Check sheet for the modelled part. Datum: model origin and axes. Units: mm. A direction names the side the tool comes from. Round coordinates to 2 decimals unless told otherwise and drop trailing zeros. Loops run counter-clockwise (first coordinate to the right, second up) from the corner with the lowest first, then second, coordinate; pieces in that order, holes last. Notation, with made-up numbers: (52, 85) -> (70, 85) arc R38 ccw to (70, 124) -> close; hole circle Ø6 at (43.25, 88). An arc over 180 degrees is marked (long way). One line per item, written item: value. Start each with the question number.
1. Material ranges on L1, parallel to X at y = 11, z = 5.75; L2, parallel to Y at x = -0.5, z = 4.5; L3, parallel to Y at x = 56, z = 0.75, recorded low to high.
2. Set-up check for faces 4 (the face through (-49.01, -42.45, 3.22)), 5 (the face through (-117.614, -82.61, 3.219)): record each of +Z, -Z, +X, -X, +Y, -Y from which the full face is reachable in a straight line by a thin tool's end or side.
3. Release check for a two-part mould opening along Y. For faces 1 (the face through (-16.45, 53.61, 3.22)), 2 (the face through (-117.614, 82.61, 3.219)), 3 (the face through (117.535, -82.689, 3.219)) record: +Y half, -Y half, draft (parallel to the pull), parting line (faces both ways), or undercut.
4. Cross-section at C-C on y = 50.5. Record the cut outline in (x, z).
5. Cross-section at B-B on x = -54.5. Record the cut outline in (y, z), then the cut area to 3 significant figures.
6. Cross-section at A-A on z = 5.25. Record the cut outline in (x, y) (1 decimal), then the cut area to 3 significant figures.
from build123d import *

# Parameters (mm, degrees)
F0_W     = 238.125
F0_H     = 168.275
F1_DEPTH = 6.35
F2_R     = 5.08
F4_DEPTH = 25.4
F5_DEPTH = 6.351
F7_DEPTH = 6.351


with BuildPart() as f1:
    # F0 (on Top) → F1 (new body)
    with BuildSketch(Plane.XY):
        Rectangle(F0_W, F0_H)
    extrude(amount=F1_DEPTH)

    # F2
    f2_edges = [f1.edges().sort_by_distance(p)[0] for p in [
        (-119.0625, 84.1375, 3.175),
        (119.0625, 84.1375, 3.175),
        (-119.0625, -84.1375, 3.175),
        (119.0625, -84.1375, 3.175),
    ]]
    fillet(f2_edges, radius=F2_R)

    # F3 (on face) → F4 (cut)
    with BuildSketch(Plane.XY.offset(6.35)):
        Polygon((-63.5, -58.7375), (0, -58.7375), (63.5, -58.7375), (31.75, -26.9875), (31.75, 36.5125), (0, 68.2625), (-31.75, 36.5125), (-31.75, -26.9875), align=None)
    extrude(amount=-F4_DEPTH, mode=Mode.SUBTRACT)

    # F3 (on face) → F5 (cut, through all)
    with BuildSketch(Plane.XY.offset(6.35)):
        Polygon((-63.5, -58.7375), (0, -58.7375), (63.5, -58.7375), (31.75, -26.9875), (31.75, 36.5125), (0, 68.2625), (-31.75, 36.5125), (-31.75, -26.9875), align=None)
    extrude(amount=-F5_DEPTH, mode=Mode.SUBTRACT)

    # F6 (on face) → F7 (cut, through all)
    with BuildSketch(Plane.XY.offset(6.35)):
        with BuildLine():
            Line((-33.02, 36.712399), (-33.02, -26.135297))
            ThreePointArc((-33.02, -26.135297), (-33.079937, -26.436622), (-33.250624, -26.692073))
            Line((-33.250624, -26.692073), (-65.221875, -58.663324))
            ThreePointArc((-65.221875, -58.663324), (-65.392562, -59.521425), (-64.665099, -60.0075))
            Line((-64.665099, -60.0075), (64.665099, -60.0075))
            ThreePointArc((64.665099, -60.0075), (65.392562, -59.521425), (65.221875, -58.663324))
            Line((65.221875, -58.663324), (33.250624, -26.692073))
            ThreePointArc((33.250624, -26.692073), (33.079937, -26.436622), (33.02, -26.135297))
            Line((33.02, -26.135297), (33.02, 36.712399))
            ThreePointArc((33.02, 36.712399), (32.960063, 37.013724), (32.789376, 37.269175))
            Line((32.789376, 37.269175), (0.556776, 69.501775))
            ThreePointArc((0.556776, 69.501775), (0, 69.732399), (-0.556776, 69.501775))
            Line((-0.556776, 69.501775), (-32.789376, 37.269175))
            ThreePointArc((-32.789376, 37.269175), (-32.960063, 37.013724), (-33.02, 36.712399))
        make_face()
    extrude(amount=-F7_DEPTH, mode=Mode.SUBTRACT)


solid = f1.part
Taken from the geometry:
1. L1: x = -119.06 to -33.02, 33.02 to 119.06
1. L2: y = -84.14 to -60.01, 69.55 to 84.14
1. L3: y = -84.14 to -60.01, -49.44 to 84.14
2. face 4: +Z, -Z
2. face 5: +Z, -Z, -X, -Y
3. face 1: undercut
3. face 2: +Y half
3. face 3: -Y half
4. outline: (-119.06, 0) -> (-19.56, 0) -> (-19.56, 6.35) -> (-119.06, 6.35) -> close; (19.56, 0) -> (119.06, 0) -> (119.06, 6.35) -> (19.56, 6.35) -> close
5. outline: (-84.14, 0) -> (-60.01, 0) -> (-60.01, 6.35) -> (-84.14, 6.35) -> close; (-47.94, 0) -> (84.14, 0) -> (84.14, 6.35) -> (-47.94, 6.35) -> close
5. area: 992 mm2
6. outline: (-119.1, -79.1) arc R5.1 ccw to (-114, -84.1) -> (114, -84.1) arc R5.1 ccw to (119.1, -79.1) -> (119.1, 79.1) arc R5.1 ccw to (114, 84.1) -> (-114, 84.1) arc R5.1 ccw to (-119.1, 79.1) -> close; hole (-65.2, -58.7) arc R0.8 ccw to (-64.7, -60) -> (64.7, -60) arc R0.8 ccw to (65.2, -58.7) -> (33.3, -26.7) arc R0.8 cw to (33, -26.1) -> (33, 36.7) arc R0.8 ccw to (32.8, 37.3) -> (0.6, 69.5) arc R0.8 ccw to (-0.6, 69.5) -> (-32.8, 37.3) arc R0.8 ccw to (-33, 36.7) -> (-33, -26.1) arc R0.8 cw to (-33.3, -26.7) -> close
6. area: 31,400 mm2
